Can you work these out from the model? Positions are in its coordinate system, mm. Face numbers are marked on the shaded views. Give positions to 0.01 mm unless a question says otherwise; leave off trailing zeros. Order: outer loops, then holes, each group sorted by start corner. A loop starts at its lowest first (then second) coordinate and runs counter-clockwise, first axis right, second up. Notation, with made-up numbers: (44.5, -7.75) -> (81.5, -7.75) arc R25 ccw to (81.5, 18.25) -> close; hole circle Ø10 at (70, -5.75). An arc over 180 degrees is marked (long way). Answer as a JSON object with one key per item and string values.
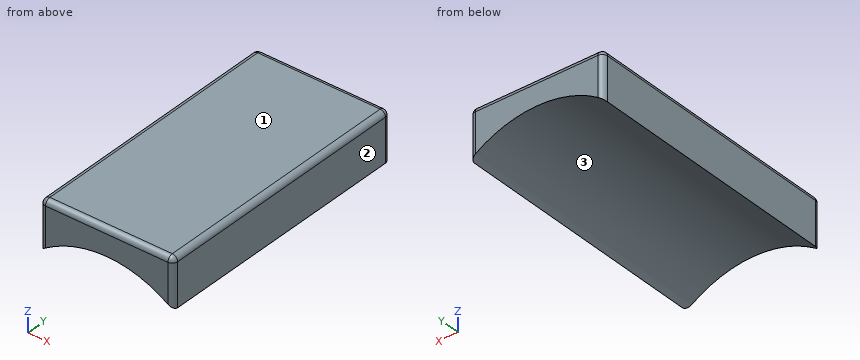
```python
from build123d import *

# Parameters (mm, degrees)
F1_DEPTH = 50
F2_R     = 1


with BuildPart() as f1:
    # F0 (on Front) → F1 (new body)
    with BuildSketch(Plane.XZ):
        with BuildLine():
            Line((12.5, 26), (-12.5, 26))
            Line((-12.5, 26), (-12.5, 16.874537))
            ThreePointArc((-12.5, 16.874537), (0, 21.04193), (12.5, 16.874537))
            Line((12.5, 16.874537), (12.5, 26))
        make_face()
    extrude(amount=F1_DEPTH)

    # F2
    f2_edges = [f1.edges().sort_by_distance(p)[0] for p in [
        (12.5, -25, 26),
        (-12.5, -25, 26),
        (0, 0, 26),
        (0, -50, 26),
        (12.5, -50, 21.437269),
        (-12.5, -50, 21.437269),
        (-12.5, 0, 21.437269),
        (12.5, 0, 21.437269),
    ]]
    fillet(f2_edges, radius=F2_R)


solid = f1.part
```
1. If we mould it in two halves opening along X, with no side actions, what happens to the marked faces 1, 2 and 3? For each: +X half, -X half, draft (parallel to the pull), parting line (faces both ways), or undercut.
Worked answers:
{"face 1": "draft", "face 2": "+X half", "face 3": "undercut"}
2. Please list where these lines run through material, in increasing order: L1, parallel to X at y = -13.5, z = 17.75; L2, parallel to X at y = -20, z = 18.25; L3, parallel to Z at x = 0.5, y = -40.
Worked answers:
{"L1": "-12.5 to -11.24, 11.24 to 12.5", "L2": "-12.5 to -10.42, 10.42 to 12.5", "L3": "21.04 to 26"}
3. If we section it at B-B on z = 18.5: Please give me the cut outline in (x, y).
Worked answers:
{"outline": "(-12.5, -49) arc R1 ccw to (-11.5, -50) -> (-9.97, -50) -> (-9.97, 0) -> (-11.5, 0) arc R1 ccw to (-12.5, -1) -> close; (9.97, -50) -> (11.5, -50) arc R1 ccw to (12.5, -49) -> (12.5, -1) arc R1 ccw to (11.5, 0) -> (9.97, 0) -> close"}
4. If we section it at A-A on y = -18: Please give me the cut outline in (x, z), then the cut area to 3 significant figures.
Worked answers:
{"outline": "(-12.5, 16.87) arc R20.83 cw to (12.5, 16.87) -> (12.5, 25) arc R1 ccw to (11.5, 26) -> (-11.5, 26) arc R1 ccw to (-12.5, 25) -> close", "area": "157 mm²"}
5. If we section it at C-C on x = -0.25: Please give me the cut outline in (y, z).
Worked answers:
{"outline": "(-50, 21.04) -> (0, 21.04) -> (0, 25) arc R1 ccw to (-1, 26) -> (-49, 26) arc R1 ccw to (-50, 25) -> close"}
6. Will these pins go through, and if not, where does the flat tip stop? pin 1 Ø6 at (x, y) = (4.5, -34.5) entering from -Z; pin 2 Ø2 at (x, z) = (-10, 19.5) entering from +Y; pin 3 Ø1.5 at (x, y) = (-8, -44.5) entering from -Z.
Worked answers:
{"pin 1": "z = 19.64", "pin 2": "y = 0", "pin 3": "z = 19.12"}
